from build123d import *


with BuildPart() as part:
    # Эскиз1 → Повернуть1 (revolve)
    with BuildSketch(Plane.XY):
        Polygon((5.024077793, 22.7), (5.102689462, 24.2), (11.15, 24.2), (11.15, 25.2), (5.155097241, 25.2), (5.23370891, 26.7), (11.15, 26.7), (11.15, 27.7), (5.286116689, 27.7), (5.364728358, 29.2), (11.15, 29.2), (11.15, 30.2), (5.417136137, 30.2), (5.495747806, 31.7), (11.15, 31.7), (11.15, 32.7), (5.548155586, 32.7), (5.626767255, 34.2), (11.15, 34.2), (11.15, 35.2), (5.679175034, 35.2), (5.757786703, 36.7), (11.15, 36.7), (11.15, 37.7), (5.810194482, 37.7), (5.888806151, 39.2), (11.15, 39.2), (11.15, 40.2), (5.94121393, 40.2), (6.019825599, 41.7), (11.15, 41.7), (11.15, 42.7), (2.5, 42.7), (2.5, 24.8), (2.1, 24.559655752), (2.1, 12.7), (3.25, 12.7), (3.25, 9.7), (2.1, 9.7), (2.1, 0), (8, 0), (8, 3.7), (6, 3.7), (6, 9.7), (8, 9.7), (8, 12.7), (4.5, 12.7), (4.578611669, 14.2), (8, 14.2), (8, 15.2), (4.631019448, 15.2), (4.709631117, 16.7), (11.15, 16.7), (11.15, 17.7), (4.762038896, 17.7), (4.840650565, 19.2), (11.15, 19.2), (11.15, 20.2), (4.893058345, 20.2), (4.971670014, 21.7), (11.15, 21.7), (11.15, 22.7), align=None)
    revolve(axis=Axis((0, 42.7, 0), (0, -1, 0)))


solid = part.part
Could you check a few things on this model? Use its own coordinates, in mm. A direction names the side the tool comes from. Coordinates: 2 decimals unless noted, no trailing zeros. Order: outer loops, then holes, each group sorted by start corner. A loop starts at its lowest first (then second) coordinate and runs counter-clockwise, first axis right, second up. Notation, with made-up numbers: (-8.75, -14) -> (46.25, -14) arc R13 ccw to (46.25, 7) -> close; hole circle Ø11 at (-36.5, 15.25). An arc over 180 degrees is marked (long way). One line per item, written item: value. Start each with the question number.
1) Imagine slicing it at B-B on x = -9. Count the separate pieces of the cut face and the enclosed holes in it, plus the area to 3 significant figures.
2) We'd pull the mould along Z, two halves only. Please class faces 1 (the conical face through (-1.18, 30.63, -5.31)), 2 (the cylindrical face through (2.003, 18.547, 0.631)), 3 (the flat face through (0.77, 12.7, -2.12)), 4 (the flat face through (-5, 32.7, 3)): +Z half, -Z half, draft (parallel to the pull), parting line (faces both ways), or undercut.
3) Which directions (+Z, -Z, +X, -X, +Y, -Y) give clear straight access to the entire face, cutting with the end or side of a thin tool? Please do faces 5 (the cylindrical face through (10.635, 24.707, 3.349)), 6 (the conical face through (4.783, 25.627, -1.983)), 7 (the cylindrical face through (-1.73, 11.22, -7.81)).
4) I'm going to push flat-ended pins straight in: pin 1 (3 mm diameter, centred on y = 19, z = 2, fed in from +X); pin 2 (5 mm diameter, centred on y = 17, z = -6, fed in from +X); pin 3 (6 mm diameter, centred on x = -3.5, y = 9, fed in from -Z). Where does each tip first touch, or does it pass through?
5) If I drill on L1, parallel to Z at x = 0, y = 11; L2, parallel to Z at x = 0, y = 30; L3, parallel to Y at x = -2, z = -1.75, over which ranges is the centre line in solid material (lowest first)? Write a range as [from, to].
6) Imagine slicing it at A-A on y = 11.5. List the corners of the cut face in (x, z) for me.
Answer list:
1. separate pieces: 11
1. enclosed holes: 0
1. area: 145 mm2
2. face 1: parting line
2. face 2: undercut
2. face 3: undercut
2. face 4: draft
3. face 5: +Y, -Y
3. face 6: none
3. face 7: -Y
4. pin 1: stops at x = 11.14
4. pin 2: stops at x = 10.59
4. pin 3: stops at z = -7.98
5. L1: z = [-8, -3.25], [3.25, 8]
5. L2: z = [-11.15, -2.5], [2.5, 11.15]
5. L3: y = [0, 9.7], [12.7, 42.7]
6. outline: circle Ø16 at (0, 0); hole circle Ø6.5 at (0, 0)
